```python
from build123d import *

# Parameters (mm, degrees)
CROQUIS1_R                 = 1.5
SALIENTE_EXTRUIR1_DEPTH    = 2
CORTAR_EXTRUIR1_DEPTH      = 96.880459427
CORTAR_EXTRUIR1_DEPTH_BACK = 2


with BuildPart() as part:
    # Croquis1 → Saliente-Extruir1 (new body)
    with BuildSketch(Plane.XY):
        with BuildLine():
            Line((-17, 93.75), (17, 93.75))
            ThreePointArc((17, 93.75), (19.121320344, 92.871320344), (20, 90.75))
            Line((20, 90.75), (20, -73.25))
            ThreePointArc((20, -73.25), (19.121320344, -75.371320344), (17, -76.25))
            Line((17, -76.25), (-17, -76.25))
            ThreePointArc((-17, -76.25), (-19.121320344, -75.371320344), (-20, -73.25))
            Line((-20, -73.25), (-20, 90.75))
            ThreePointArc((-20, 90.75), (-19.121320344, 92.871320344), (-17, 93.75))
        make_face()
        with Locations((-16, 89.25)):
            Circle(CROQUIS1_R, mode=Mode.SUBTRACT)
        with Locations((16, 89.25)):
            Circle(CROQUIS1_R, mode=Mode.SUBTRACT)
        with Locations((-16, 40.25)):
            Circle(CROQUIS1_R, mode=Mode.SUBTRACT)
        with Locations((16, 40.25)):
            Circle(CROQUIS1_R, mode=Mode.SUBTRACT)
        with Locations((-16, -11.75)):
            Circle(CROQUIS1_R, mode=Mode.SUBTRACT)
        with Locations((16, -11.75)):
            Circle(CROQUIS1_R, mode=Mode.SUBTRACT)
        with Locations((-16, -71.75)):
            Circle(CROQUIS1_R, mode=Mode.SUBTRACT)
        with Locations((16, -71.75)):
            Circle(CROQUIS1_R, mode=Mode.SUBTRACT)
    extrude(amount=SALIENTE_EXTRUIR1_DEPTH)

    # Croquis2 → Cortar-Extruir1 (cut, two sides: drawn at the far end of the back side and taken through both)
    with BuildSketch(Plane.XY.offset(2).offset(-CORTAR_EXTRUIR1_DEPTH_BACK)):
        with BuildLine():
            Line((12.400415076, 93.75), (-12.400415076, 93.75))
            ThreePointArc((-12.400415076, 93.75), (-11.253262204, 93.388304089), (-10.521029835, 92.434040287))
            Line((-10.521029835, 92.434040287), (-7.839267822, 85.065959713))
            ThreePointArc((-7.839267822, 85.065959713), (-7.107035454, 84.111695911), (-5.959882581, 83.75))
            Line((-5.959882581, 83.75), (5.959882581, 83.75))
            ThreePointArc((5.959882581, 83.75), (7.107035454, 84.111695911), (7.839267822, 85.065959713))
            Line((7.839267822, 85.065959713), (10.521029835, 92.434040287))
            ThreePointArc((10.521029835, 92.434040287), (11.253262204, 93.388304089), (12.400415076, 93.75))
        make_face()
        with BuildLine():
            ThreePointArc((-10.42045304, -27.2582672), (-12.566783681, -26.329827013), (-14, -28.177698054))
            Line((-14, -28.177698054), (-14, -54.668198657))
            ThreePointArc((-14, -54.668198657), (-12.530480645, -56.525016119), (-10.385708563, -55.521417127))
            Line((-10.385708563, -55.521417127), (-3.44772031, -41.64544062))
            ThreePointArc((-3.44772031, -41.64544062), (-3.246669118, -40.754834791), (-3.482464787, -39.872791296))
            Line((-3.482464787, -39.872791296), (-10.42045304, -27.2582672))
        make_face()
        with BuildLine():
            Line((10.42045304, -27.2582672), (3.482464787, -39.872791296))
            ThreePointArc((3.482464787, -39.872791296), (3.246669118, -40.754834791), (3.44772031, -41.64544062))
            Line((3.44772031, -41.64544062), (10.385708563, -55.521417127))
            ThreePointArc((10.385708563, -55.521417127), (12.530480645, -56.525016119), (14, -54.668198657))
            Line((14, -54.668198657), (14, -28.177698054))
            ThreePointArc((14, -28.177698054), (12.566783681, -26.329827013), (10.42045304, -27.2582672))
        make_face()
        with BuildLine():
            ThreePointArc((-4.385566091, -19.91383123), (-6.02782811, -20.850663459), (-6.057258554, -22.741116582))
            Line((-6.057258554, -22.741116582), (-1.671692462, -30.714873112))
            ThreePointArc((-1.671692462, -30.714873112), (0, -31.703296755), (1.671692462, -30.714873112))
            Line((1.671692462, -30.714873112), (6.057258554, -22.741116582))
            ThreePointArc((6.057258554, -22.741116582), (6.02782811, -20.850663459), (4.385566091, -19.91383123))
            Line((4.385566091, -19.91383123), (-4.385566091, -19.91383123))
        make_face()
        with BuildLine():
            Line((-4.385566091, -61.58616877), (4.385566091, -61.58616877))
            ThreePointArc((4.385566091, -61.58616877), (6.02782811, -60.649336541), (6.057258554, -58.758883418))
            Line((6.057258554, -58.758883418), (1.671692462, -50.785126888))
            ThreePointArc((1.671692462, -50.785126888), (0, -49.796703245), (-1.671692462, -50.785126888))
            Line((-1.671692462, -50.785126888), (-6.057258554, -58.758883418))
            ThreePointArc((-6.057258554, -58.758883418), (-6.02782811, -60.649336541), (-4.385566091, -61.58616877))
        make_face()
        with BuildLine():
            ThreePointArc((-10.42045304, 27.905564031), (-12.566783681, 28.834004217), (-14, 26.986133176))
            Line((-14, 26.986133176), (-14, 0.495632573))
            ThreePointArc((-14, 0.495632573), (-12.530480645, -1.361184889), (-10.385708563, -0.357585897))
            Line((-10.385708563, -0.357585897), (-3.44772031, 13.51839061))
            ThreePointArc((-3.44772031, 13.51839061), (-3.246669118, 14.408996439), (-3.482464787, 15.291039934))
            Line((-3.482464787, 15.291039934), (-10.42045304, 27.905564031))
        make_face()
        with BuildLine():
            Line((10.42045304, 27.905564031), (3.482464787, 15.291039934))
            ThreePointArc((3.482464787, 15.291039934), (3.246669118, 14.408996439), (3.44772031, 13.51839061))
            Line((3.44772031, 13.51839061), (10.385708563, -0.357585897))
            ThreePointArc((10.385708563, -0.357585897), (12.530480645, -1.361184889), (14, 0.495632573))
            Line((14, 0.495632573), (14, 26.986133176))
            ThreePointArc((14, 26.986133176), (12.566783681, 28.834004217), (10.42045304, 27.905564031))
        make_face()
        with BuildLine():
            ThreePointArc((-4.385566091, 35.25), (-6.02782811, 34.313167771), (-6.057258554, 32.422714648))
            Line((-6.057258554, 32.422714648), (-1.671692462, 24.448958118))
            ThreePointArc((-1.671692462, 24.448958118), (0, 23.460534475), (1.671692462, 24.448958118))
            Line((1.671692462, 24.448958118), (6.057258554, 32.422714648))
            ThreePointArc((6.057258554, 32.422714648), (6.02782811, 34.313167771), (4.385566091, 35.25))
            Line((4.385566091, 35.25), (-4.385566091, 35.25))
        make_face()
        with BuildLine():
            Line((-4.385566091, -6.42233754), (4.385566091, -6.42233754))
            ThreePointArc((4.385566091, -6.42233754), (6.02782811, -5.485505311), (6.057258554, -3.595052188))
            Line((6.057258554, -3.595052188), (1.671692462, 4.378704342))
            ThreePointArc((1.671692462, 4.378704342), (0, 5.367127985), (-1.671692462, 4.378704342))
            Line((-1.671692462, 4.378704342), (-6.057258554, -3.595052188))
            ThreePointArc((-6.057258554, -3.595052188), (-6.02782811, -5.485505311), (-4.385566091, -6.42233754))
        make_face()
        with BuildLine():
            ThreePointArc((-10.42045304, 78.905564031), (-12.566783681, 79.834004217), (-14, 77.986133176))
            Line((-14, 77.986133176), (-14, 51.495632573))
            ThreePointArc((-14, 51.495632573), (-12.530480645, 49.638815111), (-10.385708563, 50.642414103))
            Line((-10.385708563, 50.642414103), (-3.44772031, 64.51839061))
            ThreePointArc((-3.44772031, 64.51839061), (-3.246669118, 65.408996439), (-3.482464787, 66.291039934))
            Line((-3.482464787, 66.291039934), (-10.42045304, 78.905564031))
        make_face()
        with BuildLine():
            Line((10.42045304, 78.905564031), (3.482464787, 66.291039934))
            ThreePointArc((3.482464787, 66.291039934), (3.246669118, 65.408996439), (3.44772031, 64.51839061))
            Line((3.44772031, 64.51839061), (10.385708563, 50.642414103))
            ThreePointArc((10.385708563, 50.642414103), (12.530480645, 49.638815111), (14, 51.495632573))
            Line((14, 51.495632573), (14, 77.986133176))
            ThreePointArc((14, 77.986133176), (12.566783681, 79.834004217), (10.42045304, 78.905564031))
        make_face()
        with BuildLine():
            Line((-4.385566091, 44.57766246), (4.385566091, 44.57766246))
            ThreePointArc((4.385566091, 44.57766246), (6.02782811, 45.514494689), (6.057258554, 47.404947812))
            Line((6.057258554, 47.404947812), (1.671692462, 55.378704342))
            ThreePointArc((1.671692462, 55.378704342), (0, 56.367127985), (-1.671692462, 55.378704342))
            Line((-1.671692462, 55.378704342), (-6.057258554, 47.404947812))
            ThreePointArc((-6.057258554, 47.404947812), (-6.02782811, 45.514494689), (-4.385566091, 44.57766246))
        make_face()
    extrude(amount=CORTAR_EXTRUIR1_DEPTH + CORTAR_EXTRUIR1_DEPTH_BACK, mode=Mode.SUBTRACT)


solid = part.part
```
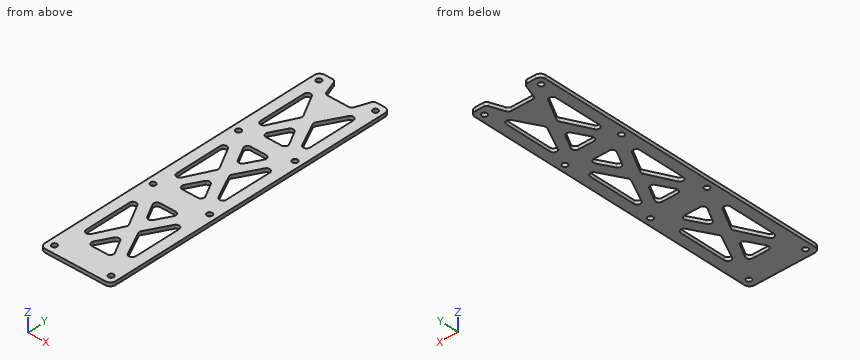
Verification items for the finished model (mm, model axes). Round coordinates to 2 decimals unless told otherwise and drop trailing zeros. Write each loop counter-clockwise with the first axis right and the second up, starting at its lowest first coordinate (ties: lowest second). Pieces come first, ordered by that corner, then holes.
1. Section check C-C on z = 1.25. State how many separate pieces and enclosed holes the cut face has, plus the area to 3 significant figures.
2. Section check D-D on y = 7. Enter the section's corners in (x, z), plus the area to 3 significant figures.
3. Section check A-A on y = -71.75. Enter the section's corners in (x, z).
4. Scan lines: L1, parallel to Y at x = 16, z = 0.65; L2, parallel to X at y = 14.5, z = 0.9; L3, parallel to X at y = 89.25, z = 1. Record each from-to range of solid material in increasing order.
5. Gauge pin test, flat ends, axial feed: P1, Ø4, axis at x = 16, y = -11.75, coming from the +Z side; P2, Ø1, axis at x = 0.5, z = 0.5, coming from the +Y side; P3, Ø1, axis at x = 11, z = 1.5, coming from the +Y side; P4, Ø1.8, axis at x = -16, y = -11.75, coming from the -Z side. Record the tip position at first contact, or that the pin passes through.
6. Section check B-B on y = 89.25. Enter the section's corners in (x, z), plus the area to 3 significant figures.
Answer:
1. separate pieces: 1
1. enclosed holes: 19
1. area: 4,800 mm2
2. outline: (-20, 0) - (-14, 0) - (-14, 2) - (-20, 2) - close; (-6.71, 0) - (6.71, 0) - (6.71, 2) - (-6.71, 2) - close; (14, 0) - (20, 0) - (20, 2) - (14, 2) - close
2. area: 50.8 mm2
3. outline: (-20, 0) - (-17.5, 0) - (-17.5, 2) - (-20, 2) - close; (-14.5, 0) - (14.5, 0) - (14.5, 2) - (-14.5, 2) - close; (17.5, 0) - (20, 0) - (20, 2) - (17.5, 2) - close
4. L1: y = -76.25 to -73.25, -70.25 to -13.25, -10.25 to 38.75, 41.75 to 87.75, 90.75 to 93.75
4. L2: x = -20 to -14, -3.25 to 3.25, 14 to 20
4. L3: x = -20 to -17.5, -14.5 to -9.36, 9.36 to 14.5, 17.5 to 20
5. P1: stops at z = 2
5. P2: stops at y = 83.75
5. P3: stops at y = 93.54
5. P4: passes through
6. outline: (-20, 0) - (-17.5, 0) - (-17.5, 2) - (-20, 2) - close; (-14.5, 0) - (-9.36, 0) - (-9.36, 2) - (-14.5, 2) - close; (9.36, 0) - (14.5, 0) - (14.5, 2) - (9.36, 2) - close; (17.5, 0) - (20, 0) - (20, 2) - (17.5, 2) - close
6. area: 30.6 mm2
